For this review, use the dimensioned drawing (mm, ordinates from the lowest corner) and the shaded views. A direction names the side the tool comes from. Coordinates: 2 decimals unless noted, no trailing zeros. Write each loop counter-clockwise with the first axis right and the second up, starting at its lowest first coordinate (ties: lowest second). Pieces come first, ordered by that corner, then holes. Notation, with made-up numbers: (79, 44) - (112, 44) arc R8 ccw to (112, 56) - close; hole circle Ø2 at (79.25, -21.5). An arc over 180 degrees is marked (long way). Answer as a JSON object with one key per item and string values.
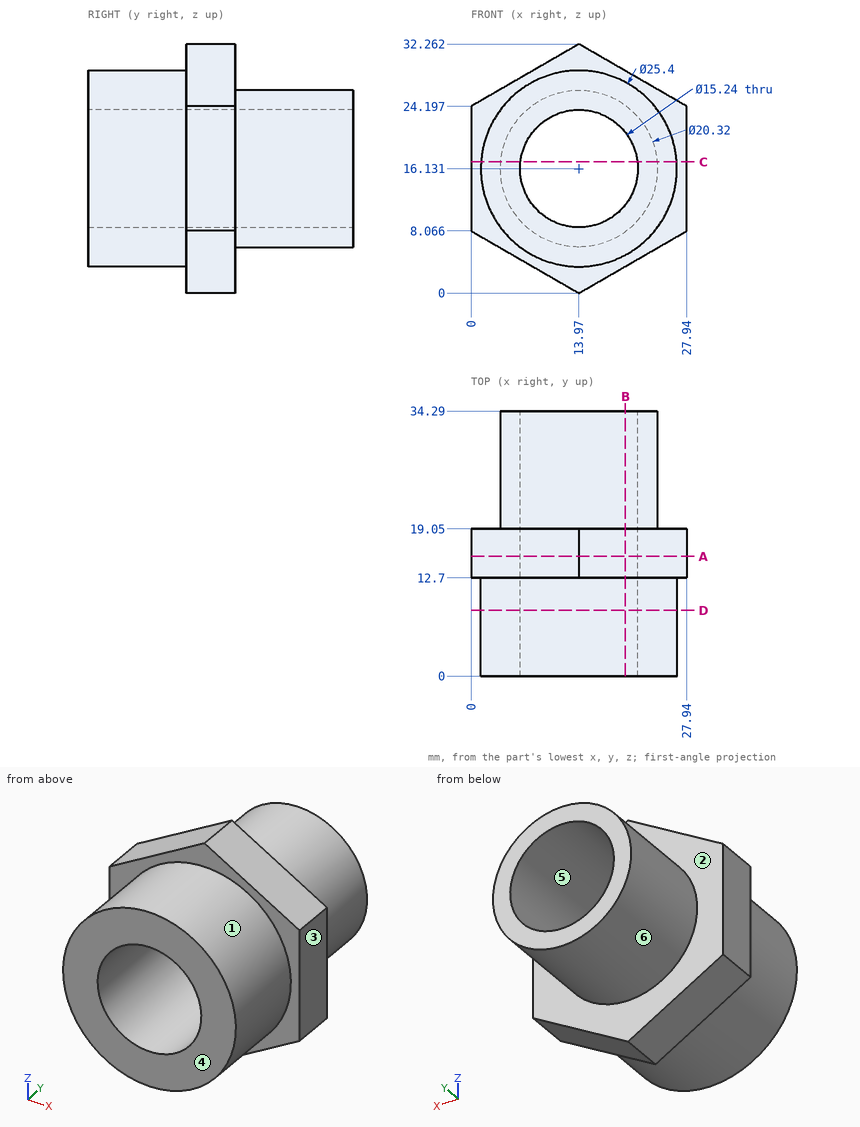
(1) Tool access review of the marked faces 1, 2 and 3: name each direction out of +Z, -Z, +X, -X, +Y, -Y from which nothing blocks a thin tool from reaching the whole face with its end or side.
Solved:
{"face 1": "-Y", "face 2": "+Y", "face 3": "+Z, -Z, +X, +Y, -Y"}
(2) Take a section at B-B, the plane x = 20. Write out the cut boundary in (y, z).
Solved:
{"outline": "(0, 4.95) - (12.7, 4.95) - (12.7, 3.48) - (19.05, 3.48) - (19.05, 7.95) - (34.29, 7.95) - (34.29, 11.47) - (0, 11.47) - close; (0, 20.79) - (34.29, 20.79) - (34.29, 24.31) - (19.05, 24.31) - (19.05, 28.78) - (12.7, 28.78) - (12.7, 27.31) - (0, 27.31) - close"}
(3) The part is to be moulded in two halves that separate along Z. For the marked faces 4, 5 and 6, say which applies: pulls with the +Z half, pulls with the -Z half, needs draft (parallel to the pull), parting line crosses it, or undercut.
Solved:
{"face 4": "needs draft", "face 5": "undercut", "face 6": "parting line crosses it"}
(4) Take a section at A-A, the plane y = 15.5. Write out the cut boundary in (x, z) (1 decimal).
Solved:
{"outline": "(0, 8.1) - (14, 0) - (27.9, 8.1) - (27.9, 24.2) - (14, 32.3) - (0, 24.2) - close; hole circle Ø15.2 at (14, 16.1)"}
(5) Take a section at C-C, the plane z = 17. Write out the cut boundary in (x, y).
Solved:
{"outline": "(0, 12.7) - (1.3, 12.7) - (1.3, 0) - (6.4, 0) - (6.4, 34.29) - (3.85, 34.29) - (3.85, 19.05) - (0, 19.05) - close; (21.54, 0) - (26.64, 0) - (26.64, 12.7) - (27.94, 12.7) - (27.94, 19.05) - (24.09, 19.05) - (24.09, 34.29) - (21.54, 34.29) - close"}
(6) Take a section at D-D, the plane y = 8.5. Write out the cut boundary in (x, z).
Solved:
{"outline": "circle Ø25.4 at (13.97, 16.13); hole circle Ø15.24 at (13.97, 16.13)"}
(7) For pin 1 (2 mm diameter, centred on x = 13.5, y = 10, fed in from +Z); pin 2 (2 mm diameter, centred on x = 17.5, y = 28.5, fed in from +Z); pin 3 (10 mm diameter, centred on x = 8.5, y = 15, fed in from +Z), all flat-tipped, find the tip position at first contact; note any pin that passes through.
Solved:
{"pin 1": "stops at z = 28.83", "pin 2": "stops at z = 25.97", "pin 3": "stops at z = 31.99"}
(8) To check wall thickness, follow line 1 (Y direction, x = 21, z = 24); line 2 (Y direction, x = 9, z = 4); line 3 (Z direction, x = 19, y = 26) (1 decimal). State the ranges of each line that lie inside material, in increasing order. Write a range as from..to.
Solved:
{"line 1": "y = 0..19.05", "line 2": "y = 12.7..19.05", "line 3": "z = 7.3..10.4, 21.9..25"}
